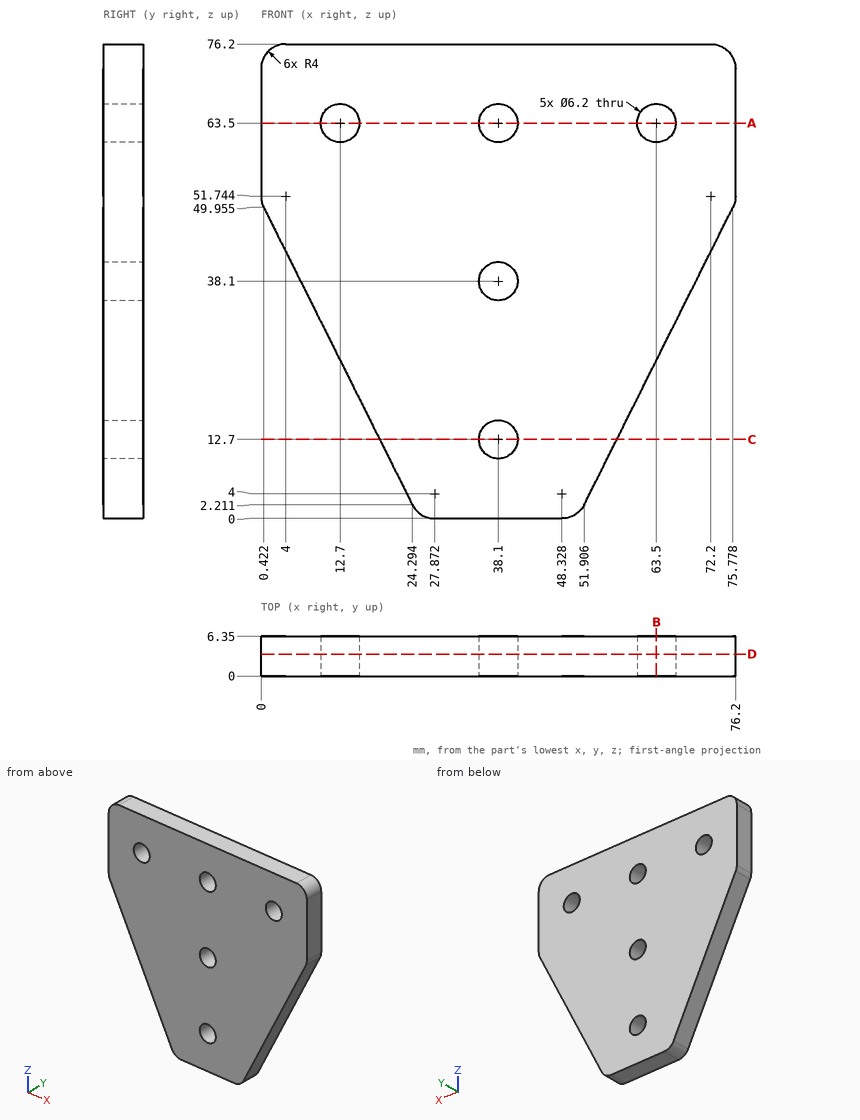
Geometry: see drawing. Coordinates: mm, zero at the bounding-box minimum. Round coordinates to 2 decimals unless told otherwise and drop trailing zeros. Write each loop counter-clockwise with the first axis right and the second up, starting at its lowest first coordinate (ties: lowest second). Pieces come first, ordered by that corner, then holes.
1) Cut plane B-B (x = 63.5). Return the cut outline in (y, z).
2) Cut plane D-D (y = 3.5). Return the cut outline in (x, z) (1 decimal), then the cut area to 3 significant figures.
3) Contact query for a flat-ended pin moving along its axis: P1, Ø5.5, axis at x = 38.1, z = 38.1, coming from the +Y side. Output: stop coordinate, or through.
4) Ray query, L1, parallel to X at y = 2, z = 63.5; L2, parallel to Z at x = 15, y = 3.5 (1 decimal); L3, parallel to X at y = 1.5, z = 66 (1 decimal). Return the intervals inside material, ascending.
5) Cut plane C-C (z = 12.7). Return the cut outline in (x, y).
6) Cut plane A-A (z = 63.5). Return the cut outline in (x, y), then the cut area to 3 significant figures.
Geometry says:
1. outline: (0, 25.4) - (6.35, 25.4) - (6.35, 60.4) - (0, 60.4) - close; (0, 66.6) - (6.35, 66.6) - (6.35, 76.2) - (0, 76.2) - close
2. outline: (0, 51.7) arc R4 ccw to (0.4, 50) - (24.3, 2.2) arc R4 ccw to (27.9, 0) - (48.3, 0) arc R4 ccw to (51.9, 2.2) - (75.8, 50) arc R4 ccw to (76.2, 51.7) - (76.2, 72.2) arc R4 ccw to (72.2, 76.2) - (4, 76.2) arc R4 ccw to (0, 72.2) - close; hole circle Ø6.2 at (12.7, 63.5); hole circle Ø6.2 at (38.1, 12.7); hole circle Ø6.2 at (38.1, 38.1); hole circle Ø6.2 at (38.1, 63.5); hole circle Ø6.2 at (63.5, 63.5)
2. area: 4,360 mm2
3. P1: passes through
4. L1: x = 0 to 9.6, 15.8 to 35, 41.2 to 60.4, 66.6 to 76.2
4. L2: z = 20.8 to 61.4, 65.6 to 76.2
4. L3: x = 0 to 10.9, 14.5 to 36.3, 39.9 to 61.7, 65.3 to 76.2
5. outline: (19.05, 0) - (35, 0) - (35, 6.35) - (19.05, 6.35) - close; (41.2, 0) - (57.15, 0) - (57.15, 6.35) - (41.2, 6.35) - close
6. outline: (0, 0) - (9.6, 0) - (9.6, 6.35) - (0, 6.35) - close; (15.8, 0) - (35, 0) - (35, 6.35) - (15.8, 6.35) - close; (41.2, 0) - (60.4, 0) - (60.4, 6.35) - (41.2, 6.35) - close; (66.6, 0) - (76.2, 0) - (76.2, 6.35) - (66.6, 6.35) - close
6. area: 366 mm2
